Could you check a few things on this model? Use its own coordinates, in mm. A direction names the side the tool comes from. Coordinates: 2 decimals unless noted, no trailing zeros. Order: outer loops, then holes, each group sorted by start corner. A loop starts at its lowest first (then second) coordinate and runs counter-clockwise, first axis right, second up. Notation, with made-up numbers: (13.5, 13.25) - (21.5, 13.25) arc R15 ccw to (21.5, 36.25) - close; hole circle Ø7 at (86, 13). An arc over 180 degrees is marked (long way). Answer as a JSON object with one key per item and string values. Group by question number.
(1) Imagine slicing it at C-C, the plane z = 11.5. Give the number of separate pieces and of enclosed holes in the cut face, and give its area (3 significant figures).
(2) Imagine slicing it at B-B, the plane y = 4.5. Write out the boundary of the cut face in (x, z), and give its area (3 significant figures).
(3) Which directions (+Z, -Z, +X, -X, +Y, -Y) give clear straight access to the entire face, cutting with the end or side of a thin tool? Please do faces 1 (the cylindrical face through (-13.017, 0.608, -11.76)), 2 (the flat face through (-2, 4, -2)).
(4) Please list where these lines run through material, in increasing order: probe 1 along X at (y, z) = (0.3, 11.5); probe 2 along X at (y, z) = (0.45, -11.5); probe 3 along X at (y, z) = (1.25, -8).
(5) We'd pull the mould along X, two halves only. Please class faces 3 (the flat face through (0, 1, -16)), 4 (the cylindrical face through (16.983, 0.608, 11.24)), 5 (the flat face through (19, 1, 0)): pulls with the +X half, pulls with the -X half, needs draft (parallel to the pull), parting line crosses it, or undercut.
(6) Will these pins go through, and if not, where does the flat tip stop? P1, Ø4.5, axis at x = 15, z = 11.5, coming from the -Y side; P2, Ø6, axis at x = -0.5, z = 2.5, coming from the -Y side; P3, Ø6.5, axis at x = 15, z = -11.5, coming from the +Y side; P4, Ø1.5, axis at y = 4, z = -3, coming from the +X side.
from build123d import *

# Parameters (mm, degrees)
SKIZZE1_W                       = 38
SKIZZE1_H                       = 32
AUFSATZ_LINEAR_AUSTRAGEN1_DEPTH = 1.2
SKIZZE2_R                       = 15
AUFSATZ_LINEAR_AUSTRAGEN2_DEPTH = 5
VERRUNDUNG1_R                   = 5
SCHNITT_LINEAR_AUSTRAGEN1_REACH = 27.338
SKIZZE3_R                       = 2
SKIZZE4_R                       = 14
SCHNITT_LINEAR_AUSTRAGEN2_DEPTH = 4
VERRUNDUNG2_R                   = 4
SKIZZE5_R                       = 2.5
SCHNITT_LINEAR_AUSTRAGEN3_DEPTH = 26.601562452
VERRUNDUNG3_R                   = 4


with BuildPart() as part:
    # Skizze1 → Aufsatz-Linear austragen1 (new body)
    with BuildSketch(Plane(origin=(0, 0, 0), x_dir=(1, 0, 0), z_dir=(0, 1, 0))):
        Rectangle(SKIZZE1_W, SKIZZE1_H)
    extrude(amount=AUFSATZ_LINEAR_AUSTRAGEN1_DEPTH)

    # Skizze2 → Aufsatz-Linear austragen2 (add)
    with BuildSketch(Plane(origin=(0, 1.2, 0), x_dir=(1, 0, 0), z_dir=(0, 1, 0))):
        with Locations(Location((0, 0, 0), (0, 0, 270))):
            Circle(SKIZZE2_R)
    extrude(amount=AUFSATZ_LINEAR_AUSTRAGEN2_DEPTH)

    # Verrundung1
    verrundung1_edges = [part.edges().sort_by_distance(p)[0] for p in [
        (0, 6.2, -15),
    ]]
    fillet(verrundung1_edges, radius=VERRUNDUNG1_R - 0.0001)  # a hair under: the kernel refuses the full size

    # Skizze3 → Schnitt-Linear austragen1 (cut, up to next)
    with BuildSketch(Plane(origin=(0, 1.2, 0), x_dir=(1, 0, 0), z_dir=(0, 1, 0)), mode=Mode.PRIVATE) as schnitt_linear_austragen1_sk1:
        with Locations(Location((-15, 11.5, 0), (0, 0, 270))):
            Circle(SKIZZE3_R)
    schnitt_linear_austragen1_tool1 = extrude(schnitt_linear_austragen1_sk1.sketch, amount=-SCHNITT_LINEAR_AUSTRAGEN1_REACH, mode=Mode.PRIVATE) & part.part
    # Skizze3 → Schnitt-Linear austragen1 (cut, up to next)
    with BuildSketch(Plane(origin=(0, 1.2, 0), x_dir=(1, 0, 0), z_dir=(0, 1, 0)), mode=Mode.PRIVATE) as schnitt_linear_austragen1_sk2:
        with Locations(Location((15, 11.5, 0), (0, 0, 270))):
            Circle(SKIZZE3_R)
    schnitt_linear_austragen1_tool2 = extrude(schnitt_linear_austragen1_sk2.sketch, amount=-SCHNITT_LINEAR_AUSTRAGEN1_REACH, mode=Mode.PRIVATE) & part.part
    # Skizze3 → Schnitt-Linear austragen1 (cut, up to next)
    with BuildSketch(Plane(origin=(0, 1.2, 0), x_dir=(1, 0, 0), z_dir=(0, 1, 0)), mode=Mode.PRIVATE) as schnitt_linear_austragen1_sk3:
        with Locations(Location((15, -11.5, 0), (0, 0, 270))):
            Circle(SKIZZE3_R)
    schnitt_linear_austragen1_tool3 = extrude(schnitt_linear_austragen1_sk3.sketch, amount=-SCHNITT_LINEAR_AUSTRAGEN1_REACH, mode=Mode.PRIVATE) & part.part
    # Skizze3 → Schnitt-Linear austragen1 (cut, up to next)
    with BuildSketch(Plane(origin=(0, 1.2, 0), x_dir=(1, 0, 0), z_dir=(0, 1, 0)), mode=Mode.PRIVATE) as schnitt_linear_austragen1_sk4:
        with Locations(Location((-15, -11.5, 0), (0, 0, 270))):
            Circle(SKIZZE3_R)
    schnitt_linear_austragen1_tool4 = extrude(schnitt_linear_austragen1_sk4.sketch, amount=-SCHNITT_LINEAR_AUSTRAGEN1_REACH, mode=Mode.PRIVATE) & part.part
    add(schnitt_linear_austragen1_tool1.solids().sort_by_distance((-15, 1.2, -11.5))[0], mode=Mode.SUBTRACT)
    add(schnitt_linear_austragen1_tool2.solids().sort_by_distance((15, 1.2, -11.5))[0], mode=Mode.SUBTRACT)
    add(schnitt_linear_austragen1_tool3.solids().sort_by_distance((15, 1.2, 11.5))[0], mode=Mode.SUBTRACT)
    add(schnitt_linear_austragen1_tool4.solids().sort_by_distance((-15, 1.2, 11.5))[0], mode=Mode.SUBTRACT)

    # Skizze4 → Schnitt-Linear austragen2 (cut)
    with BuildSketch(Plane.XZ):
        with Locations(Location((0, 0, 0), (0, 0, 270))):
            Circle(SKIZZE4_R)
    extrude(amount=-SCHNITT_LINEAR_AUSTRAGEN2_DEPTH, mode=Mode.SUBTRACT)

    # Verrundung2
    verrundung2_edges = [part.edges().sort_by_distance(p)[0] for p in [
        (0, 4, 14),
    ]]
    fillet(verrundung2_edges, radius=VERRUNDUNG2_R - 0.0001)  # a hair under: the kernel refuses the full size

    # Skizze5 → Schnitt-Linear austragen3 (cut, through all)
    with BuildSketch(Plane(origin=(0, 6.2, 0), x_dir=(1, 0, 0), z_dir=(0, 1, 0))):
        with Locations(Location((0, 0, 0), (0, 0, 270))):
            Circle(SKIZZE5_R)
    extrude(amount=-SCHNITT_LINEAR_AUSTRAGEN3_DEPTH, mode=Mode.SUBTRACT)

    # Verrundung3
    verrundung3_edges = [part.edges().sort_by_distance(p)[0] for p in [
        (19, 0.6, 16),
        (-19, 0.6, 16),
        (-19, 0.6, -16),
        (19, 0.6, -16),
    ]]
    fillet(verrundung3_edges, radius=VERRUNDUNG3_R)


solid = part.part
Result set:
{
 "1": {"separate pieces": "3", "enclosed holes": "0", "area": "63.2 mm^2"},
 "2": {"outline": "circle Ø27.51 at (0, 0); hole circle Ø5 at (0, 0)", "area": "575 mm^2"},
 "3": {"face 1": "+Y, -Y", "face 2": "-Y"},
 "4": {"probe 1": "x = -19 to -17, -13 to -7.96, 7.96 to 13, 17 to 19", "probe 2": "x = -19 to -17, -13 to -7.94, 7.94 to 13, 17 to 19", "probe 3": "x = -12.69 to -11.24, 11.24 to 12.69"},
 "5": {"face 3": "needs draft", "face 4": "undercut", "face 5": "pulls with the +X half"},
 "6": {"P1": "stops at y = 0", "P2": "stops at y = 4", "P3": "stops at y = 1.2", "P4": "stops at x = 14.28"}
}
